from build123d import *

# Parameters (mm, degrees)
SKETCH3_W           = 3
SKETCH3_H           = 5
BOSS_EXTRUDE1_DEPTH = 3
SKETCH5_R           = 4
CUT_EXTRUDE1_DEPTH  = 5


with BuildPart() as part:
    # Sketch1 → Revolve1 (revolve)
    with BuildSketch(Plane.XZ):
        Polygon((7.5, 5), (0, 5), (0, 3), (15, 3), (15, 0), (17.5, 0), (17.5, 35), (15, 35), (15, 5), (10, 5), (10, 30), (7.5, 30), align=None)
    revolve(axis=Axis((0, 0, 35), (0, 0, -1)))

    # Sketch3 → Boss-Extrude1 (add)
    with BuildSketch(Plane.XY.offset(25)):
        with Locations((-1.5, 17.5)):
            Rectangle(SKETCH3_W, SKETCH3_H)
        with Locations((-1.5, -17.5)):
            Rectangle(SKETCH3_W, SKETCH3_H)
    extrude(amount=-BOSS_EXTRUDE1_DEPTH)

    # Sketch5 → Cut-Extrude1 (cut)
    with BuildSketch(Plane(origin=(0, 13, 0), x_dir=(1, 0, 0), z_dir=(0, 1, 0))):
        with Locations((0, -10)):
            Circle(SKETCH5_R)
    extrude(amount=CUT_EXTRUDE1_DEPTH, mode=Mode.SUBTRACT)


solid = part.part
Model file for the job. Use its own axes, mm. A direction names the side the tool comes from. Coordinates: 2 decimals unless noted, no trailing zeros. Write each loop counter-clockwise with the first axis right and the second up, starting at its lowest first coordinate (ties: lowest second). Pieces come first, ordered by that corner, then holes. Notation, with made-up numbers: (-22.5, -22.75) -> (-2.5, -22.75) arc R17 ccw to (-2.5, -3.75) -> close; hole circle Ø5 at (-19.75, 36). An arc over 180 degrees is marked (long way). One line per item, written item: value. Start each with the question number.
1) Slice it at A-A on z = 10. Write the cut outline in (x, y), then the cut area to 3 significant figures.
2) Which spindle directions (+Z, -Z, +X, -X, +Y, -Y) get a long thin tool onto all of the face, cutting with end or side? Do faces 5 (the face through (-3, 19, 24)), 6 (the face through (0, 0, 3)), 7 (the face through (0, 19, 24)). Say none if no direction does.
3) Slice it at C-C on y = 0. Write the cut outline in (x, z), then the cut area to 3 significant figures.
4) Probe probe 1 along X at (y, z) = (0, 18); probe 2 along Y at (x, z) = (0, 13); probe 3 along Y at (x, z) = (6.5, 5.5). List the from-to ranges inside material, lowest first.
5) Flat gauge pins, fed straight in: pin 1 Ø0.8 at (x, y) = (-2, 18.5) entering from +Z; pin 2 Ø5 at (x, y) = (-11.5, -0.5) entering from +Z; pin 3 Ø5 at (x, z) = (12, 31) entering from +Y. Where does each tip first touch, or does it go through?
6) Slice it at D-D on z = 20. Write the cut outline in (x, y).
7) Pull direction Z, two halves, no side cores. Call faces 1 (the face through (-7.493, -0.33, 17.325)), 2 (the face through (3.695, 15.957, 11.532)), 3 (the face through (-2, -19, 22)), 4 (the face through (4, -7, 30)): +Z half, -Z half, draft (parallel to the pull), parting line (faces both ways), or undercut.
Answers follow:
1. outline: circle Ø20 at (0, 0); (-4, 14.46) -> (-4, 17.04) arc R17.5 ccw (long way) to (4, 17.04) -> (4, 14.46) arc R15 cw (long way) to start; hole circle Ø15 at (0, 0)
1. area: 372 mm2
2. face 5: +Z, -Z, -X, +Y
2. face 6: -Z
2. face 7: +Z, -Z, +X, +Y
3. outline: (-17.5, 0) -> (-15, 0) -> (-15, 3) -> (15, 3) -> (15, 0) -> (17.5, 0) -> (17.5, 35) -> (15, 35) -> (15, 5) -> (10, 5) -> (10, 30) -> (7.5, 30) -> (7.5, 5) -> (-7.5, 5) -> (-7.5, 30) -> (-10, 30) -> (-10, 5) -> (-15, 5) -> (-15, 35) -> (-17.5, 35) -> close
3. area: 360 mm2
4. probe 1: -17.5 to -15, -10 to -7.5, 7.5 to 10, 15 to 17.5
4. probe 2: -17.5 to -15, -10 to -7.5, 7.5 to 10
4. probe 3: -16.25 to -13.52, -7.6 to -3.74, 3.74 to 7.6, 13.52 to 16.25
5. pin 1: z = 25
5. pin 2: z = 30
5. pin 3: y = 14.7
6. outline: circle Ø35 at (0, 0); circle Ø20 at (0, 0); hole circle Ø30 at (0, 0); hole circle Ø15 at (0, 0)
7. face 1: draft
7. face 2: undercut
7. face 3: -Z half
7. face 4: +Z half
